Here's how the part is built. I have some questions about the finished solid (model axes, mm). A direction names the side the tool comes from. Coordinates: 2 decimals unless noted, no trailing zeros. Loops run counter-clockwise (first coordinate to the right, second up) from the corner with the lowest first, then second, coordinate; pieces in that order, holes last. Notation, with made-up numbers: M -6.75,61 L 29.25,61 A18 cw 29.25,78 Z; hole C 60.25,64 d8. An arc over 180 degrees is marked long. Use one line per item in the form item = value. Start each with the question number.
(1) Imagine slicing it at B-B, the plane x = 15.5. Please give me the cut outline in (y, z).
(2) Imagine slicing it at C-C, the plane z = 1.85. State how many separate pieces and enclosed holes the cut face has, and give its area (3 significant figures).
(3) Thinking about a two-plate mould opening in Y: for faces 1 (the flat face through (-75, -43.25, 1)), 2 (the cylindrical face through (-84.11, -72.32, 1.48)), 3 (the flat face through (-68.56, -69, 2)), 4 (the flat face through (38.878, -37, 1)), which applies, +Y half, -Y half, draft (parallel to the pull), parting line (faces both ways), or undercut?
(4) Please list where these lines run through material, in increasing order: L1, parallel to X at y = -41, z = 2.15; L2, parallel to Y at x = -17.5, z = 0.45; L3, parallel to X at y = -30, z = 1.3.
(5) On a 3-axis mill with a long thin cutter (end or side, diameter ignored), from which of +Z, -Z, +X, -X, +Y, -Y can I reach the whole of each face in a straight line? I mean faces 5 (the flat face through (-4, -43.25, 1)), 6 (the flat face through (44.878, -37, 1)), 7 (the flat face through (53.878, -37, 1)). Say none if no direction works.
(6) Imagine slicing it at A-A, the plane y = -34. Please give me the cut outline in (x, z), and give its area (3 significant figures).
(7) Will these pins go through, and if not, where does the flat tip stop? P1, Ø1.5, axis at x = -70, z = 2, coming from the +Y side; P2, Ø1.5, axis at y = -35, z = 2, coming from the -X side; P3, Ø0.9, axis at y = -36, z = 1.5, coming from the +X side.
(8) Imagine slicing it at D-D, the plane x = 51.5. Please give me the cut outline in (y, z).
```python
from build123d import *

# Parameters (mm, degrees)
BOSS_EXTRUDE1_DEPTH = 3
FILLET2_R           = 5
SKETCH2_W           = 129.874983815
SKETCH2_H           = 3
CUT_EXTRUDE1_DEPTH  = 10


with BuildPart() as part:
    # Sketch1 → Boss-Extrude1 (new body)
    with BuildSketch(Plane.XY):
        with BuildLine():
            Line((-88.622208542, -43.25), (-61.122208542, -43.25))
            Line((-61.122208542, -43.25), (-61.122208542, -26.25))
            Line((-61.122208542, -26.25), (-46.122208542, -26.25))
            Line((-46.122208542, -26.25), (-46.122208542, -43.25))
            Line((-46.122208542, -43.25), (38.877791458, -43.25))
            Line((38.877791458, -43.25), (38.877791458, -26.25))
            Line((38.877791458, -26.25), (53.877791458, -26.25))
            Line((53.877791458, -26.25), (53.877791458, -43.25))
            Line((53.877791458, -43.25), (81.377791458, -43.25))
            Line((81.377791458, -43.25), (81.377791458, -61.598486101))
            ThreePointArc((81.377791458, -61.598486101), (76.984393176, -72.205087819), (66.377791458, -76.598486101))
            Line((66.377791458, -76.598486101), (-73.622208542, -76.598486101))
            ThreePointArc((-73.622208542, -76.598486101), (-84.228810259, -72.205087819), (-88.622208542, -61.598486101))
            Line((-88.622208542, -61.598486101), (-88.622208542, -43.25))
        make_face()
        with BuildLine():
            Line((-55.122208542, -43.25), (-55.122208542, -30.75))
            ThreePointArc((-55.122208542, -30.75), (-53.622208542, -29.25), (-52.122208542, -30.75))
            Line((-52.122208542, -30.75), (-52.122208542, -43.25))
            ThreePointArc((-52.122208542, -43.25), (-53.622208542, -44.75), (-55.122208542, -43.25))
        make_face(mode=Mode.SUBTRACT)
        with BuildLine():
            Line((44.877791458, -43.25), (44.877791458, -30.75))
            ThreePointArc((44.877791458, -30.75), (46.377791458, -29.25), (47.877791458, -30.75))
            Line((47.877791458, -30.75), (47.877791458, -43.25))
            ThreePointArc((47.877791458, -43.25), (46.377791458, -44.75), (44.877791458, -43.25))
        make_face(mode=Mode.SUBTRACT)
    extrude(amount=BOSS_EXTRUDE1_DEPTH)

    # Fillet2
    fillet2_edges = [part.edges().sort_by_distance(p)[0] for p in [
        (-61.122208542, -26.25, 1.5),
        (-46.122208542, -26.25, 1.5),
        (38.877791458, -26.25, 1.5),
        (53.877791458, -26.25, 1.5),
    ]]
    fillet(fillet2_edges, radius=FILLET2_R)

    # Sketch2 → Cut-Extrude1 (cut)
    with BuildSketch(Plane.XY.offset(3)):
        with Locations((-3.622208542, -69.098486101)):
            Rectangle(SKETCH2_W, SKETCH2_H)
    extrude(amount=-CUT_EXTRUDE1_DEPTH, mode=Mode.SUBTRACT)


solid = part.part
```
Answer:
q1.outline = M -76.6,0 L -70.6,0 L -70.6,3 L -76.6,3 Z; M -67.6,0 L -43.25,0 L -43.25,3 L -67.6,3 Z
q2.separate_pieces = 1
q2.enclosed_holes = 3
q2.area = 5,580 mm²
q3.face_1 = +Y half
q3.face_2 = -Y half
q3.face_3 = undercut
q3.face_4 = draft
q4.L1 = -61.12 to -55.12, -52.12 to -46.12, 38.88 to 44.88, 47.88 to 53.88
q4.L2 = -76.6 to -70.6, -67.6 to -43.25
q4.L3 = -60.96 to -54.92, -52.32 to -46.28, 39.04 to 45.08, 47.68 to 53.72
q5.face_5 = +Z, -Z, +Y
q5.face_6 = +Z, -Z
q5.face_7 = +Z, -Z, +X, +Y
q6.outline = M -61.12,0 L -55.12,0 L -55.12,3 L -61.12,3 Z; M -52.12,0 L -46.12,0 L -46.12,3 L -52.12,3 Z; M 38.88,0 L 44.88,0 L 44.88,3 L 38.88,3 Z; M 47.88,0 L 53.88,0 L 53.88,3 L 47.88,3 Z
q6.area = 72.0 mm²
q7.P1 = -43.25
q7.P2 = -61.12
q7.P3 = 53.88
q8.outline = M -76.6,0 L -70.6,0 L -70.6,3 L -76.6,3 Z; M -67.6,0 L -26.99,0 L -26.99,3 L -67.6,3 Z
